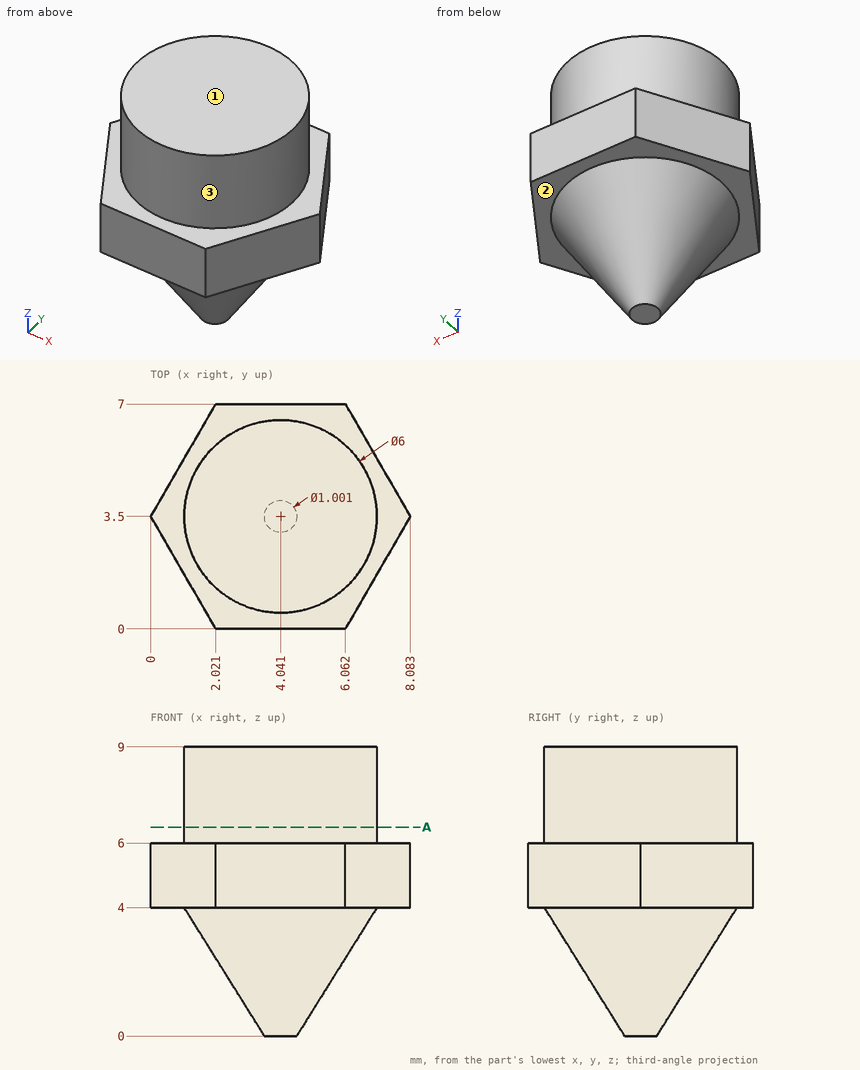
Check sheet for the drawn part. Datum: minimum x, y, z corner. Units: mm. A direction names the side the tool comes from. Give positions to 0.01 mm unless a question says otherwise; leave off trailing zeros. Loops run counter-clockwise (first coordinate to the right, second up) from the corner with the lowest first, then second, coordinate; pieces in that order, holes last. Notation, with made-up numbers: M 22,11 L 36,11 A12 ccw 36,26 Z; hole C 87.5,52.5 d4. An arc over 180 degrees is marked long. Answer as CSV lines item,"result".
Item 1: Set-up check for the marked faces 1, 2 and 3: record each of +Z, -Z, +X, -X, +Y, -Y from which the full face is reachable in a straight line by a thin tool's end or side.
Reply:
face 1,"+Z, +X, -X, +Y, -Y"
face 2,"-Z"
face 3,"+Z"
Item 2: Sectioned sample at A-A, the plane z = 6.5. Enter the section's corners in (x, y), then the cut area to 3 significant figures.
Reply:
outline,"C 4.04,3.5 d6"
area,"28.3 mm^2"
Item 3: Scan lines: L1, parallel to Z at x = 1.5, y = 5.5; L2, parallel to X at y = 5.5, z = 4.75 (1 decimal); L3, parallel to X at y = 6, z = 4.5 (1 decimal). Record each from-to range of solid material in increasing order.
Reply:
L1,"4 to 6"
L2,"1.2 to 6.9"
L3,"1.4 to 6.6"
